Can you work these out from the model? Positions are in its coordinate system, mm. A direction names the side the tool comes from. Give positions to 0.01 mm unless a question says otherwise; leave off trailing zeros. Write each loop counter-clockwise with the first axis right and the second up, starting at its lowest first coordinate (ties: lowest second). Pieces come first, ordered by that corner, then holes.
from build123d import *
from build123d import SkipClean  # not in build123d's __all__

# Parameters (mm, degrees)
F1_DEPTH      = 6
F2_R          = 22.5
F3_DEPTH      = 3
F3_DEPTH_BACK = 12


with BuildPart() as f1:
    # F0 (on Front) → F1 (new body)
    with BuildSketch(Plane.XZ):
        with BuildLine():
            ThreePointArc((-15.9360760742, 39.4846993069), (-19.545554777, 42.911846885), (-24.5, 42.4352447854))
            ThreePointArc((-24.5, 42.4352447854), (-29.1533569815, 39.3837755518), (-33.430729205, 35.824381988))
            ThreePointArc((-33.430729205, 35.824381988), (-35.3334015022, 31.2250869161), (-33.1097213112, 26.7721189803))
            Line((-33.1097213112, 26.7721189803), (-24.5775940866, 19.8731444143))
            ThreePointArc((-24.5775940866, 19.8731444143), (-22.8056864044, 16.8994131973), (-23.3899197808, 13.487462795))
            ThreePointArc((-23.3899197808, 13.487462795), (-26.8258933187, -3.0612820274), (-19.7498381023, -18.410428972))
            ThreePointArc((-19.7498381023, -18.410428972), (-18.4119152904, -21.6030292813), (-19.4682866758, -24.8995143308))
            Line((-19.4682866758, -24.8995143308), (-26.2267146235, -33.5433963703))
            ThreePointArc((-26.2267146235, -33.5433963703), (-27.3899721372, -38.3828704105), (-24.5, -42.4352447854))
            ThreePointArc((-24.5, -42.4352447854), (-19.530671634, -44.9394355274), (-14.3094602739, -46.8640517526))
            ThreePointArc((-14.3094602739, -46.8640517526), (-9.3750177536, -46.212166761), (-6.6304744945, -42.0599192579))
            Line((-6.6304744945, -42.0599192579), (-4.9218508726, -31.2213930501))
            ThreePointArc((-4.9218508726, -31.2213930501), (-3.2324779357, -28.2000103756), (0.0144744773, -26.9999961202))
            ThreePointArc((0.0144744773, -26.9999961202), (16.0640946633, -21.7012640795), (25.8188182355, -7.8986470313))
            ThreePointArc((25.8188182355, -7.8986470313), (27.9147298015, -5.1436717332), (31.2977552903, -4.410273664))
            Line((31.2977552903, -4.410273664), (42.1627906977, -5.9413029366))
            ThreePointArc((42.1627906977, -5.9413029366), (46.9355269143, -4.5289764745), (49, 0))
            ThreePointArc((49, 0), (48.6840286155, 5.5556599757), (47.740189479, 11.0396697646))
            ThreePointArc((47.740189479, 11.0396697646), (44.7084192558, 14.987079845), (39.7401958057, 15.2878002776))
            Line((39.7401958057, 15.2878002776), (29.4994449592, 11.3482486357))
            ThreePointArc((29.4994449592, 11.3482486357), (26.0381643401, 11.3005971783), (23.3754453035, 13.5125333252))
            ThreePointArc((23.3754453035, 13.5125333252), (10.7617986555, 24.7625461069), (-6.0689801331, 26.3090760032))
            ThreePointArc((-6.0689801331, 26.3090760032), (-9.5028145111, 26.7467010144), (-11.8294686145, 29.3097879948))
            Line((-11.8294686145, 29.3097879948), (-15.9360760742, 39.4846993069))
        make_face()
        with BuildLine():
            ThreePointArc((-18.2977896407, -42.3131291004), (-18.3599561093, -42.3518337374), (-18.4225903326, -42.3897767579))
            ThreePointArc((-18.4225903326, -42.3897767579), (-18.4375826284, -42.3180972643), (-18.4516989687, -42.2462401305))
            ThreePointArc((-18.4516989687, -42.2462401305), (-20.7833159026, -41.1492865077), (-23.05, -39.9237711145))
            ThreePointArc((-23.05, -39.9237711145), (-24.1846787517, -35.6890923627), (-19.95, -34.554413611))
            ThreePointArc((-19.95, -34.554413611), (-18.1421434856, -35.5369192496), (-16.2860412235, -36.4249208821))
            ThreePointArc((-16.2860412235, -36.4249208821), (-15.9677964631, -36.1891617461), (-15.6346911323, -35.9749120408))
            ThreePointArc((-15.6346911323, -35.9749120408), (-15.5640668297, -36.3646225815), (-15.519307053, -36.7581434324))
            ThreePointArc((-15.519307053, -36.7581434324), (-13.6037364042, -37.5093102555), (-11.6519890802, -38.1607278557))
            ThreePointArc((-11.6519890802, -38.1607278557), (-9.5924128846, -42.0308888206), (-13.4625738495, -44.0904650162))
            ThreePointArc((-13.4625738495, -44.0904650162), (-15.9050276013, -43.2693898386), (-18.2977896407, -42.3131291004))
        make_face(mode=Mode.SUBTRACT)
        with BuildLine():
            ThreePointArc((2.0410607887, 4.9020578186), (3.3561252192, 4.1149147638), (4.3915942436, 2.9849623113))
            ThreePointArc((4.3915942436, 2.9849623113), (5.3099999882, 0.0003538209), (4.3919919982, -2.9843770351))
            ThreePointArc((4.3919919982, -2.9843770351), (3.4698827698, -4.0194543864), (2.3112879445, -4.7805907624))
            Line((2.3112879445, -4.7805907624), (1.2434795246, -12.010568624))
            ThreePointArc((1.2434795246, -12.010568624), (-2.1944705259, -14.838607263), (-4.6609590448, -11.1327015059))
            Line((-4.6609590448, -11.1327015059), (-3.6838317901, -4.5167128251))
            Line((-3.6838317901, -4.5167128251), (-3.5940513986, -3.9088226545))
            ThreePointArc((-3.5940513986, -3.9088226545), (-5.0887135619, -1.5169358209), (-5.1476659417, 1.3029333647))
            ThreePointArc((-5.1476659417, 1.3029333647), (-4.6350123617, 2.5908995362), (-3.8064652091, 3.7022861332))
            ThreePointArc((-3.8064652091, 3.7022861332), (-1.0672517117, 5.2016414509), (2.0410607887, 4.9020578186))
        make_face(mode=Mode.SUBTRACT)
        with BuildLine():
            ThreePointArc((-23.05, 39.9237711145), (-18.8153212483, 38.7890923627), (-19.95, 34.554413611))
            ThreePointArc((-19.95, 34.554413611), (-21.7048030996, 33.4800167624), (-23.401886203, 32.3165858677))
            ThreePointArc((-23.401886203, 32.3165858677), (-23.3568351823, 31.9230982526), (-23.3378421601, 31.5274957213))
            ThreePointArc((-23.3378421601, 31.5274957213), (-23.7106535397, 31.6611885515), (-24.0738324819, 31.8191858732))
            ThreePointArc((-24.0738324819, 31.8191858732), (-25.6821473576, 30.5358364402), (-27.2221652098, 29.1712824759))
            ThreePointArc((-27.2221652098, 29.1712824759), (-31.60361102, 29.322717652), (-31.4521758439, 33.7041634621))
            ThreePointArc((-31.4521758439, 33.7041634621), (-29.5198770058, 35.4088528699), (-27.4953498942, 37.0029152121))
            ThreePointArc((-27.4953498942, 37.0029152121), (-27.4977858588, 37.0761052717), (-27.4993283668, 37.1493196105))
            ThreePointArc((-27.4993283668, 37.1493196105), (-27.4297559565, 37.1264635728), (-27.3604676831, 37.1027601152))
            ThreePointArc((-27.3604676831, 37.1027601152), (-25.244669512, 38.5735228004), (-23.05, 39.9237711145))
        make_face(mode=Mode.SUBTRACT)
        with BuildLine():
            ThreePointArc((45.7931395349, 5.3102138882), (45.8577419681, 5.2757284657), (45.9219186994, 5.2404571474))
            ThreePointArc((45.9219186994, 5.2404571474), (45.8673385849, 5.1916336916), (45.8121666518, 5.1434800154))
            ThreePointArc((45.8121666518, 5.1434800154), (46.0279854146, 2.5757637074), (46.1, 0))
            ThreePointArc((46.1, 0), (43, -3.1), (39.9, 0))
            ThreePointArc((39.9, 0), (39.8469465851, 2.0569024872), (39.6879274265, 4.1083350144))
            ThreePointArc((39.6879274265, 4.1083350144), (39.3246316454, 4.2660634935), (38.9725332924, 4.4474163195))
            ThreePointArc((38.9725332924, 4.4474163195), (39.2747203695, 4.70343403), (39.5931395349, 4.9389575592))
            ThreePointArc((39.5931395349, 4.9389575592), (39.2858837618, 6.9734738153), (38.87415429, 8.9894453798))
            ThreePointArc((38.87415429, 8.9894453798), (41.1960239046, 12.7081711687), (44.9147496935, 10.3863015541))
            ThreePointArc((44.9147496935, 10.3863015541), (45.4249046071, 7.8605369687), (45.7931395349, 5.3102138882))
        make_face(mode=Mode.SUBTRACT)
    extrude(amount=F1_DEPTH)

    # F2 (on face) → F3 (join, two sides)
    with BuildSketch(Plane.XZ.offset(6)) as f3_sk:
        Circle(F2_R)
        with BuildLine():
            Line((-4.6609590448, -11.1327015059), (-3.5940513986, -3.9088226545))
            ThreePointArc((-3.5940513986, -3.9088226545), (0.7754775485, 5.2530690621), (2.3112879445, -4.7805907624))
            Line((2.3112879445, -4.7805907624), (1.2434795246, -12.010568624))
            ThreePointArc((1.2434795246, -12.010568624), (-2.1944705259, -14.838607263), (-4.6609590448, -11.1327015059))
        make_face(mode=Mode.SUBTRACT)
    with SkipClean():  # cleaning this boolean's faces spoils the solid; the shape is the same uncleaned
        extrude(amount=F3_DEPTH)
        extrude(f3_sk.sketch, amount=-F3_DEPTH_BACK)


solid = f1.part
(1) Imagine slicing it at A-A, the plane y = 4.25. Write out the boundary of the cut face in (x, z).
Returned:
outline: circle Ø45 at (0, 0); hole (-4.66, -11.13) arc R3 ccw (long way) to (1.24, -12.01) - (2.31, -4.78) arc R5.31 ccw (long way) to (-3.59, -3.91) - close
(2) Imagine slicing it at D-D, the plane y = -5. Give the number of separate pieces and of enclosed holes in the cut face, plus the area to 3 significant figures.
Returned:
separate pieces: 1
enclosed holes: 4
area: 3,110 mm2
(3) Will these pins go through, and if not, where does the flat tip stop? P1, Ø3, axis at x = 30.5, y = -1, coming from the -Z side; P2, Ø4, axis at x = -26.5, z = -9.5, coming from the +Y side; P3, Ø12, axis at x = 3, z = 29, coming from the -Y side.
Returned:
P1: stops at z = -4.62
P2: stops at y = 0
P3: stops at y = -6
(4) For faces 1 (the face through (7, -6, 22)), 2 (the face through (-25.66, -2.958, 30.554)), 3 (the face through (-22.8, -2.96, -29.16)), which set-ups out of +Z, -Z, +X, -X, +Y, -Y let a thin tool reach every point of the face, with its end or its side?
Returned:
face 1: -Y
face 2: +Y, -Y
face 3: -X, +Y, -Y
(5) Imagine slicing it at B-B, the plane z = 7. Write out the boundary of the cut face in (x, y).
Returned:
outline: (-26.08, -6) - (-21.38, -6) - (-21.38, -9) - (21.38, -9) - (21.38, -6) - (39.28, -6) - (39.28, 0) - (21.38, 0) - (21.38, 6) - (-21.38, 6) - (-21.38, 0) - (-26.08, 0) - close; (45.57, -6) - (48.5, -6) - (48.5, 0) - (45.57, 0) - close
(6) Imagine slicing it at C-C, the plane x = -21.5. Write out the boundary of the cut face in (y, z).
Returned:
outline: (-9, -6.63) - (-6, -6.63) - (-6, -16.33) - (0, -16.33) - (0, -6.63) - (6, -6.63) - (6, 6.63) - (0, 6.63) - (0, 33.61) - (-6, 33.61) - (-6, 6.63) - (-9, 6.63) - close; (-6, -44.03) - (0, -44.03) - (0, -40.78) - (-6, -40.78) - close; (-6, -34.14) - (0, -34.14) - (0, -27.5) - (-6, -27.5) - close; (-6, 40.34) - (0, 40.34) - (0, 43.24) - (-6, 43.24) - close
(7) If we mould it in two halves opening along Z, with no side actions, what happens to faces 4 (the face through (10.382, -7.479, -19.961)), 5 (the face through (5, -9, -5)), 6 (the face through (-2.12, -1.39, -14.85))? For each: +Z half, -Z half, draft (parallel to the pull), parting line (faces both ways), or undercut.
Returned:
face 4: parting line
face 5: draft
face 6: undercut
(8) If I drill on L1, parallel to X at y = -0.5, z = 2; L2, parallel to Z at x = 0, y = -1.5; L3, parallel to Z at x = 0, y = 0.5, over which ranges is the centre line in solid material (lowest first)?
Returned:
L1: x = -26.93 to -4.92, 4.92 to 39.85, 46.06 to 48.96
L2: z = -27 to -14.31, 5.31 to 27
L3: z = -22.5 to -14.31, 5.31 to 22.5
